```python
from build123d import *

# Parameters (mm, degrees)
F0_R     = 400
F1_DEPTH = 30
F3_R     = 25
F4_DEPTH = 0.1
F5_R     = 17.5
F6_DEPTH = 60


with BuildPart() as f1:
    # F0 (on Top) → F1 (new body)
    with BuildSketch(Plane.XY):
        Circle(F0_R)
    extrude(amount=F1_DEPTH)

    # F3 (on face) → F4 (join)
    with BuildSketch(Plane.XY.offset(30)):
        with Locations((212.132034, 212.132034)):
            Circle(F3_R)
        with Locations((212.132034, -212.132034)):
            Circle(F3_R)
        with Locations((-212.132034, -212.132034)):
            Circle(F3_R)
        with Locations((-212.132034, 212.132034)):
            Circle(F3_R)
        with Locations((0, 150)):
            Circle(F3_R)
        with Locations((0, -150)):
            Circle(F3_R)
        with Locations((150, 0)):
            Circle(F3_R)
        with Locations((-150, 0)):
            Circle(F3_R)
        with Locations((0, 300)):
            Circle(F3_R)
        with Locations((300, 0)):
            Circle(F3_R)
        with Locations((0, -300)):
            Circle(F3_R)
        with Locations((-300, 0)):
            Circle(F3_R)
    extrude(amount=F4_DEPTH)

    # F5 (on face) → F6 (cut)
    with BuildSketch(Plane.XY.offset(30)):
        Circle(F5_R)
    extrude(amount=-F6_DEPTH, mode=Mode.SUBTRACT)


solid = f1.part
```
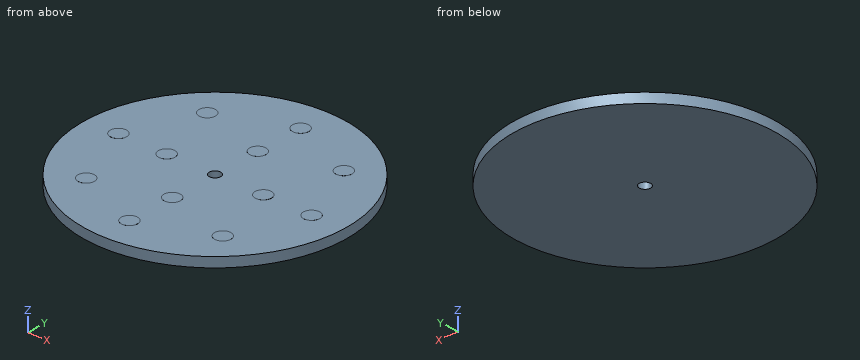
For this review, take the finished solid that the model builds, in its own axes (mm). Coordinates: 2 decimals unless noted, no trailing zeros. Loops run counter-clockwise (first coordinate to the right, second up) from the corner with the lowest first, then second, coordinate; pieces in that order, holes last.
1. Add section C-C, the plane z = 11. Give the boundary of the cut face in (x, y), then the cut area to 3 significant figures.
2. Add section A-A, the plane y = 0. Give the boundary of the cut face in (x, z).
3. Insertion check: P1, Ø8, axis at x = 284.5, z = 9, coming from the +Y side; P2, Ø4, axis at y = -53.5, z = 11.5, coming from the -X side; P3, Ø1, axis at x = 90, z = 11.5, coming from the +Y side. Each pin has a flat end and moves straight along its axis. Give the tip position at first contact, or say it passes through.
4. For line 1 (Y direction, x = 0, z = 21.75); line 2 (Z direction, x = 16.5, y = 361.5); line 3 (Y direction, x = 4, z = 26), list the stretches that pass through material, from the lowest coordinate up.
5. Add section D-D, the plane y = 150. Give the boundary of the cut face in (x, z), then the cut area to 3 significant figures.
Result:
1. outline: circle Ø800 at (0, 0); hole circle Ø35 at (0, 0)
1. area: 502,000 mm2
2. outline: (-400, 0) - (-17.5, 0) - (-17.5, 30) - (-125, 30) - (-125, 30.1) - (-175, 30.1) - (-175, 30) - (-275, 30) - (-275, 30.1) - (-325, 30.1) - (-325, 30) - (-400, 30) - close; (17.5, 0) - (400, 0) - (400, 30) - (325, 30) - (325, 30.1) - (275, 30.1) - (275, 30) - (175, 30) - (175, 30.1) - (125, 30.1) - (125, 30) - (17.5, 30) - close
3. P1: stops at y = 285.17
3. P2: stops at x = -396.67
3. P3: stops at y = 389.86
4. line 1: y = -400 to -17.5, 17.5 to 400
4. line 2: z = 0 to 30
4. line 3: y = -399.98 to -17.04, 17.04 to 399.98
5. outline: (-370.81, 0) - (370.81, 0) - (370.81, 30) - (25, 30) - (25, 30.1) - (-25, 30.1) - (-25, 30) - (-370.81, 30) - close
5. area: 22,300 mm2
